Here's how the part is built. I have some questions about the finished solid (model axes, mm). Coordinates: 2 decimals unless noted, no trailing zeros. Write each loop counter-clockwise with the first axis right and the second up, starting at its lowest first coordinate (ties: lowest second). Pieces come first, ordered by that corner, then holes. Notation, with made-up numbers: (36, -11.5) - (74, -11.5) arc R21 cw to (74, 9.5) - close; hole circle Ø9 at (12, 47.25). An arc over 180 degrees is marked (long way). Answer in a Markdown table with one row per item. Add a question column.
Item 1: If I drill on probe 1 along Y at (x, z) = (-3.5, 59); probe 2 along Y at (x, z) = (-0.5, 61); probe 3 along X at (y, z) = (5.5, 53.5), over which ranges is the centre line in solid material (lowest first)? Write a range as from..to.
Item 2: Imagine slicing it at C-C (y = 6.5). Please give me the cut outline in (x, z).
Item 3: Imagine slicing it at B-B (x = 1.5). Please give me the cut outline in (y, z).
Item 4: Imagine slicing it at A-A (z = 55.5). Please give me the cut outline in (x, y).
Autodesk Inventor part; units mm, degrees
ref_plane "YZ Plane" through (0, 0, 0) normal (1, 0, 0) x (0, 1, 0)
ref_plane "XZ Plane" through (0, 0, 0) normal (0, 1, 0) x (-1, 0, 0)
ref_plane "XY Plane" through (0, 0, 0) normal (0, 0, 1) x (1, 0, 0)
sketch "Sketch1" plane through (0, 0, 0) normal (0, 1, 0) x (-1, 0, 0)
  line L0 (5, 90) -> (-5, 90)
  line L1 (-5, 90) -> (-5, -90)
  line L2 (-5, -90) -> (5, -90)
  line L3 (5, -90) -> (5, 90)
  line L4 (5, 90) -> (-5, -90) construction
  line L5 (-5, 90) -> (5, -90) construction
  point P0 (0, 0)
  dimension "d0" = 10
  dimension "d1" = 180
extrude "Extrusion1" add sketch "Sketch1" along normal blind 10
chamfer "Chamfer1" distance 9 angle 45 1 edges at (5, 0, 0)
equation "\"BendRadius\" = Thickness"
equation "\"BendReliefWidth\" = Thickness"
equation "\"BendReliefDepth\" = 0.5 * Thickness"
equation "\"CornerReliefSize\" = 4 * Thickness"
equation "\"MinimumRemnant\" = 2 * Thickness"
equation "\"TransitionRadius\" = BendRadius"
equation "\"JacobiRadiusSize\" = BendRadius"
equation "\"GapSize\" = Thickness"
properties part number "rovny_diel_180"
Here are the results:
| question | item | result |
|---|---|---|
| 1 | probe 1 | y = 0.5..10 |
| 1 | probe 2 | y = 3.5..10 |
| 1 | probe 3 | x = -5..1.5 |
| 2 | outline | (-5, -90) - (2.5, -90) - (2.5, 90) - (-5, 90) - close |
| 3 | outline | (5.5, -90) - (10, -90) - (10, 90) - (5.5, 90) - close |
| 4 | outline | (-5, 0) - (-4, 0) - (5, 9) - (5, 10) - (-5, 10) - close |
